from build123d import *

# Parameters (mm, degrees)
SKETCH1_W           = 260
SKETCH1_H           = 198
BOSS_EXTRUDE1_DEPTH = 219
SKETCH2_W           = 240
SKETCH2_H           = 178
CUT_EXTRUDE1_DEPTH  = 209
SKETCH3_W           = 282
SKETCH3_H           = 220
SKETCH3_W_2         = 260
SKETCH3_H_2         = 198
BOSS_EXTRUDE2_DEPTH = 10
FILLET1_R           = 10
FILLET3_R           = 5
SKETCH4_R           = 2.17
SKETCH4_R_2         = 4.5
CUT_EXTRUDE3_DEPTH  = 20


with BuildPart() as part:
    # Sketch1 → Boss-Extrude1 (new body)
    with BuildSketch(Plane(origin=(0, 0, 0), x_dir=(1, 0, 0), z_dir=(0, 1, 0))):
        Rectangle(SKETCH1_W, SKETCH1_H)
    extrude(amount=BOSS_EXTRUDE1_DEPTH)

    # Sketch2 → Cut-Extrude1 (cut)
    with BuildSketch(Plane(origin=(0, 0, 0), x_dir=(1, 0, 0), z_dir=(0, 1, 0))):
        Rectangle(SKETCH2_W, SKETCH2_H)
    extrude(amount=CUT_EXTRUDE1_DEPTH, mode=Mode.SUBTRACT)

    # Sketch3 → Boss-Extrude2 (add)
    with BuildSketch(Plane(origin=(0, 0, 0), x_dir=(1, 0, 0), z_dir=(0, 1, 0))):
        Rectangle(SKETCH3_W, SKETCH3_H)
        Rectangle(SKETCH3_W_2, SKETCH3_H_2, mode=Mode.SUBTRACT)
    extrude(amount=BOSS_EXTRUDE2_DEPTH)

    # Fillet1
    fillet1_edges = [part.edges().sort_by_distance(p)[0] for p in [
        (-130, 114.5, -99),
        (130, 114.5, -99),
        (130, 114.5, 99),
        (-130, 114.5, 99),
    ]]
    fillet(fillet1_edges, radius=FILLET1_R)

    # Fillet3
    fillet3_edges = [part.edges().sort_by_distance(p)[0] for p in [
        (0, 10, -99),
        (130, 10, 0),
        (0, 10, 99),
        (-130, 10, 0),
        (127.071067812, 10, -96.071067812),
        (127.071067812, 10, 96.071067812),
        (-127.071067812, 10, -96.071067812),
        (-127.071067812, 10, 96.071067812),
    ]]
    fillet(fillet3_edges, radius=FILLET3_R)

    # Sketch4 → Cut-Extrude3 (cut)
    with BuildSketch(Plane(origin=(0, 219, 0), x_dir=(1, 0, 0), z_dir=(0, 1, 0))):
        with Locations(Location((-59, 0, 0), (0, 0, 270))):
            Circle(SKETCH4_R)
        with Locations(Location((-69.5, -18.186533479, 0), (0, 0, 270))):
            Circle(SKETCH4_R)
        with Locations(Location((-90.5, -18.186533479, 0), (0, 0, 270))):
            Circle(SKETCH4_R)
        with Locations(Location((-101, 0, 0), (0, 0, 270))):
            Circle(SKETCH4_R)
        with Locations(Location((-90.5, 18.186533479, 0), (0, 0, 270))):
            Circle(SKETCH4_R)
        with Locations(Location((-69.5, 18.186533479, 0), (0, 0, 270))):
            Circle(SKETCH4_R)
        with Locations(Location((-80, 0, 0), (0, 0, 270))):
            Circle(SKETCH4_R_2)
    extrude(amount=-CUT_EXTRUDE3_DEPTH, mode=Mode.SUBTRACT)


solid = part.part
The model under review builds one solid part; all positions refer to its coordinate system, in mm. A direction names the side the tool comes from. Give positions to 0.01 mm unless a question says otherwise; leave off trailing zeros. Loops run counter-clockwise (first coordinate to the right, second up) from the corner with the lowest first, then second, coordinate; pieces in that order, holes last. Notation, with made-up numbers: (41.5, 70.5) -> (54.5, 70.5) arc R15 cw to (54.5, 79.5) -> close; hole circle Ø4 at (57.5, 85). An arc over 180 degrees is marked (long way). Put each result on its own line as item: value. Start each with the question number.
1. For faces 5 (the face through (-11, 10, 105)), 6 (the face through (-2, 209, -1)), 7 (the face through (130, 116, 1)), list the 3-axis set-ups (+Z, -Z, +X, -X, +Y, -Y) from which the entire face can be reached by the end or side of a thin tool; tool diameter is ignored.
2. Clearance check with flat-ended pins moving along their axes: P1, Ø12, axis at x = -103, y = 23.5, coming from the -Z side; P2, Ø5, axis at y = 125.5, z = 14.5, coming from the +X side; P3, Ø5.5, axis at x = -90.5, z = 18.19, coming from the -Y side. State where each tip first meets the part, or that it passes through.
3. We need section D-D on x = 78. State the section outline as (y, z) points, then the cut area to 3 significant figures.
4. Mouldability with a two-part tool opening along X and no side actions: class faces 1 (the face through (-126.99, 118.43, -96.15)), 2 (the face through (-2, 103, -89)), 3 (the face through (-2, 116, 99)), 4 (the face through (-120, 103, 1)) as released by +X, released by -X, zero draft, split by the parting line, or undercut.
5. We need section A-A on x = -80. State the section outline as (y, z) points, then the cut area to 3 significant figures.
6. We need section C-C on z = -32. State the section outline as (x, y) points, then the cut area to 3 significant figures.
7. Wall thickness on probe 1 along Z at (x, y) = (-69, 211); probe 2 along X at (y, z) = (213.5, 0); probe 3 along Z at (x, y) = (-67, 143): over which ranges is each line inside the solid? List them lowest first.
8. We need section B-B on y = 64. State the section outline as (x, z) points, then the cut area to 3 significant figures.
Determined:
1. face 5: +Y
1. face 6: -Y
1. face 7: +Z, -Z, +X, +Y
2. P1: z = -99
2. P2: x = 130
2. P3: y = 209
3. outline: (0, -110) -> (10, -110) -> (10, -104) arc R5 cw to (15, -99) -> (219, -99) -> (219, 99) -> (15, 99) arc R5 cw to (10, 104) -> (10, 110) -> (0, 110) -> (0, 89) -> (209, 89) -> (209, -89) -> (0, -89) -> close
3. area: 6,390 mm^2
4. face 1: released by -X
4. face 2: undercut
4. face 3: zero draft
4. face 4: undercut
5. outline: (0, -110) -> (10, -110) -> (10, -104) arc R5 cw to (15, -99) -> (219, -99) -> (219, -4.5) -> (209, -4.5) -> (209, -89) -> (0, -89) -> close; (0, 89) -> (209, 89) -> (209, 4.5) -> (219, 4.5) -> (219, 99) -> (15, 99) arc R5 cw to (10, 104) -> (10, 110) -> (0, 110) -> close
5. area: 6,300 mm^2
6. outline: (-141, 0) -> (-120, 0) -> (-120, 209) -> (120, 209) -> (120, 0) -> (141, 0) -> (141, 10) -> (135, 10) arc R5 cw to (130, 15) -> (130, 219) -> (-130, 219) -> (-130, 15) arc R5 cw to (-135, 10) -> (-141, 10) -> close
6. area: 7,010 mm^2
7. probe 1: -99 to -20.3, -16.07 to 16.07, 20.3 to 99
7. probe 2: -130 to -103.17, -98.83 to -84.5, -75.5 to -61.17, -56.83 to 130
7. probe 3: -99 to -89, 89 to 99
8. outline: (-130, -89) arc R10 ccw to (-120, -99) -> (120, -99) arc R10 ccw to (130, -89) -> (130, 89) arc R10 ccw to (120, 99) -> (-120, 99) arc R10 ccw to (-130, 89) -> close; hole (-120, -89) -> (120, -89) -> (120, 89) -> (-120, 89) -> close
8. area: 8,670 mm^2
